CAD build for the part. Positions are in the model's coordinates, mm. A direction names the side the tool comes from. Coordinates: 2 decimals unless noted, no trailing zeros. Loops run counter-clockwise (first coordinate to the right, second up) from the corner with the lowest first, then second, coordinate; pieces in that order, holes last. Notation, with made-up numbers: M 44.5,-2 L 83.5,-2 A26 ccw 83.5,27 Z; hole C 39.25,9 d4. An arc over 180 degrees is marked long. Answer as a JSON object with one key per item and string values. Group by question number.
```python
from build123d import *

# Parameters (mm, degrees)
ESQUISSE1_R        = 30.5
BOSS_EXTRU_1_DEPTH = 30
ESQUISSE2_R        = 32.5
BOSS_EXTRU_2_DEPTH = 10
CHANFREIN1_SIZE    = 5
ESQUISSE6_R        = 2


with BuildPart() as part:
    # Esquisse1 → Boss.-Extru.1 (new body)
    with BuildSketch(Plane.XY):
        Circle(ESQUISSE1_R)
    extrude(amount=BOSS_EXTRU_1_DEPTH)

    # Esquisse2 → Boss.-Extru.2 (add)
    with BuildSketch(Plane(origin=(0, 0, 0), x_dir=(-1, 0, 0), z_dir=(0, 0, -1))):
        Circle(ESQUISSE2_R)
    extrude(amount=BOSS_EXTRU_2_DEPTH)

    # Chanfrein1
    chanfrein1_edges = [part.edges().sort_by_distance(p)[0] for p in [
        (-30.5, 0, 30),
    ]]
    chamfer(chanfrein1_edges, length=CHANFREIN1_SIZE)

    # Enlèvement de matière-Balayage1: sweep along a path in Esquisse7
    with BuildLine(Plane.XY.offset(10)) as enl_vement_de_mati_re_balayage1_path:
        CenterArc((0, 0), 26.0040611, 0, 360)
    # Esquisse6 → Enlèvement de matière-Balayage1 (sweep, cut)
    with BuildSketch(Plane(origin=(0, 0, 0), x_dir=(1, 0, 0), z_dir=(0, 1, 0))):
        with Locations((-29, -12.5)):
            Circle(ESQUISSE6_R)
    sweep(path=enl_vement_de_mati_re_balayage1_path.line, mode=Mode.SUBTRACT)


solid = part.part
```
Item 1: Slice it at C-C, the plane z = 9. Write the cut outline in (x, y), then the cut area to 3 significant figures.
Item 2: Tool access for faces 1 (the flat face through (0, 0, 30)), 2 (the cylindrical face through (-24.204, -18.559, 5.51)): list every direction of +Z, -Z, +X, -X, +Y, -Y with a clear straight run to the whole face (end or side of a thin tool).
Item 3: Drill centre lines: L1, parallel to Z at x = 4, y = 28; L2, parallel to X at y = -12, z = 11; L3, parallel to Z at x = 4.5, y = 27. Where is each one in solid material? Low to high. Write a range as from..to.
Item 4: Pin check, flat tips, straight feed: pin 1 (3 mm diameter, centred on y = -8.5, z = 22.5, fed in from +X); pin 2 (4 mm diameter, centred on x = 11, z = 12, fed in from +Y); pin 3 (3 mm diameter, centred on y = -1.5, z = 23, fed in from +X). Stop position of each tip, or through.
Item 5: Slice it at A-A, the plane y = 0. Write the cut outline in (x, z).
Computed:
{
 "1": {"outline": "C 0,0 d61", "area": "2,920 mm2"},
 "2": {"face 1": "+Z, +X, -X, +Y, -Y", "face 2": "+Z"},
 "3": {"L1": "-10..10.63, 14.37..27.22", "L2": "-28.04..-27.85, -24.94..24.94, 27.85..28.04", "L3": "-10..11.34, 13.66..28.13"},
 "4": {"pin 1": "x = 29.69", "pin 2": "y = 29.09", "pin 3": "x = 30.5"},
 "5": {"outline": "M -32.5,-10 L 32.5,-10 L 32.5,0 L 30.5,0 L 30.5,11.18 A2 cw long 30.5,13.82 L 30.5,25 L 25.5,30 L -25.5,30 L -30.5,25 L -30.5,13.82 A2 cw long -30.5,11.18 L -30.5,0 L -32.5,0 Z"}
}
